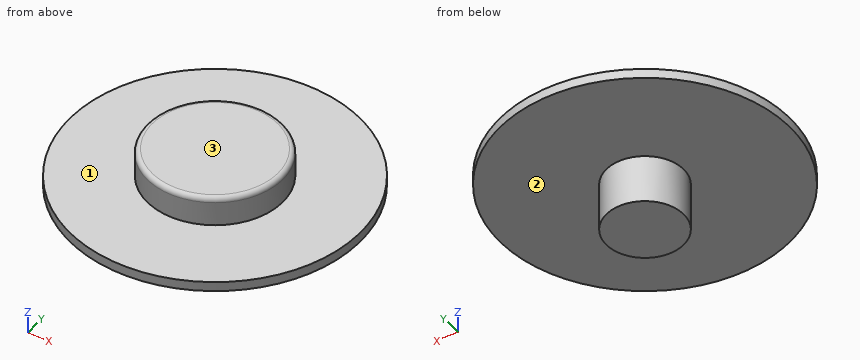
```python
from build123d import *

# Parameters (mm, degrees)
ESQUISSE1_R        = 15
BOSS_EXTRU_1_DEPTH = 1
ESQUISSE2_R        = 7
BOSS_EXTRU_2_DEPTH = 3
CONG_1_R           = 0.5
ESQUISSE3_R        = 4
BOSS_EXTRU_3_DEPTH = 5


with BuildPart() as part:
    # Esquisse1 → Boss.-Extru.1 (new body)
    with BuildSketch(Plane.XY):
        Circle(ESQUISSE1_R)
    extrude(amount=BOSS_EXTRU_1_DEPTH)

    # Esquisse2 → Boss.-Extru.2 (add)
    with BuildSketch(Plane.XY.offset(1)):
        Circle(ESQUISSE2_R)
    extrude(amount=BOSS_EXTRU_2_DEPTH)

    # Congé1
    cong_1_edges = [part.edges().sort_by_distance(p)[0] for p in [
        (-7, 0, 4),
    ]]
    fillet(cong_1_edges, radius=CONG_1_R)

    # Esquisse3 → Boss.-Extru.3 (add)
    with BuildSketch(Plane(origin=(0, 0, 0), x_dir=(-1, 0, 0), z_dir=(0, 0, -1))):
        Circle(ESQUISSE3_R)
    extrude(amount=BOSS_EXTRU_3_DEPTH)


solid = part.part
```
Can you work these out from the model? Positions are in its coordinate system, mm. Face numbers are marked on the shaded views. A direction names the side the tool comes from. Give positions to 0.01 mm unless a question says otherwise; leave off trailing zeros. Order: outer loops, then holes, each group sorted by start corner. A loop starts at its lowest first (then second) coordinate and runs counter-clockwise, first axis right, second up. Notation, with made-up numbers: M -6,52.25 L 48,52.25 A29 cw 48,74.25 Z; hole C -23.5,-35.75 d11. An arc over 180 degrees is marked long. One line per item, written item: value.
1) I want a section at A-A, the plane y = 0. List the corners of the cut face in (x, z) for me.
Answer sheet:
outline: M -15,0 L -4,0 L -4,-5 L 4,-5 L 4,0 L 15,0 L 15,1 L 7,1 L 7,3.5 A0.5 ccw 6.5,4 L -6.5,4 A0.5 ccw -7,3.5 L -7,1 L -15,1 Z
2) For P1, Ø5, axis at x = 9, z = 1, coming from the -Y side; P2, Ø15, axis at x = -4, y = -0.5, coming from the -Z side; P3, Ø4, axis at x = 2.5, z = 1.5, coming from the -Y side; P4, Ø4, axis at y = 0.5, z = -2.5, coming from the +X side, each with a flat end and sliding along its axis, tell me the tip position at first contact or that it passes through.
Answer sheet:
P1: stops at y = -13.52
P2: stops at z = -5
P3: stops at y = -14.99
P4: stops at x = 4
3) I want a section at D-D, the plane z = 2.5. List the corners of the cut face in (x, y) for me, plus the area to 3 significant figures.
Answer sheet:
outline: C 0,0 d14
area: 154 mm^2
4) On a 3-axis mill with a long thin cutter (end or side, diameter ignored), from which of +Z, -Z, +X, -X, +Y, -Y can I reach the whole of each face in a straight line? I mean the marked faces 1, 2 and 3. Say none if no direction works.
Answer sheet:
face 1: +Z
face 2: -Z
face 3: +Z, +X, -X, +Y, -Y
5) I want a section at C-C, the plane z = -2.25. List the corners of the cut face in (x, y) for me, plus the area to 3 significant figures.
Answer sheet:
outline: C 0,0 d8
area: 50.3 mm^2
6) Please list where these lines run through material, in increasing order: line 1 along Y through (x, z) = (0, 0.75); line 2 along Z through (x, y) = (-8.5, -9.5); line 3 along Z through (x, y) = (-4, -4).
Answer sheet:
line 1: y = -15 to 15
line 2: z = 0 to 1
line 3: z = 0 to 4
